Verification items for the finished model (mm, model axes). A direction names the side the tool comes from. Coordinates: 2 decimals unless noted, no trailing zeros. Write each loop counter-clockwise with the first axis right and the second up, starting at its lowest first coordinate (ties: lowest second). Pieces come first, ordered by that corner, then holes. Notation, with made-up numbers: (-39.75, 71) -> (-20.75, 71) arc R20 ccw to (-20.75, 88) -> close; hole circle Ø3 at (63, 22.25). An arc over 180 degrees is marked (long way). Use CSV: the item, a comma, the result in double quotes.
Autodesk Inventor part; units mm, degrees
ref_plane "YZ Plane" through (0, 0, 0) normal (1, 0, 0) x (0, 1, 0)
ref_plane "XZ Plane" through (0, 0, 0) normal (0, 1, 0) x (-1, 0, 0)
ref_plane "XY Plane" through (0, 0, 0) normal (0, 0, 1) x (1, 0, 0)
sketch "Sketch1 - walls" plane through (0, 0, 0) normal (0, 0, 1) x (1, 0, 0)
  line L0 (0, -9) -> (0, 9) construction
  line L1 (-10, -9) -> (-10, -12)
  line L2 (-10, -12) -> (10, -12)
  line L3 (-10, -9) -> (10, -9)
  line L4 (10, -9) -> (10, -12)
  line L5 (-10, 9) -> (10, 9)
  line L6 (10, 9) -> (10, 12)
  line L7 (10, 12) -> (-10, 12)
  line L8 (-10, 12) -> (-10, 9)
  point P0 (0, 0)
  dimension "d5" = 18
  dimension "d7" = 3
  dimension "d8" = 20
  dimension "d9" = 3
  dimension "d10" = 20
extrude "Extrusion1" add sketch "Sketch1 - walls" along normal blind 25
sketch "Sketch2 - base" plane through (0, 0, 0) normal (0, 0, -1) x (-1, 0, 0)
  circle A0 centre (0, 0) radius 18.5
  dimension "d13" = 37
sketch "Sketch3 - wall_top1" plane through (-10, 12, 25) normal (0, 1, 0) x (1, 0, 0)
  line L0 (10, 0) -> (10, -10) construction
  line L1 (20, 0) -> (0, 0)
  arc A0 (0, 0) -> (20, 0) centre (10, 0) ccw
  point P0 (10, 25)
  dimension "d16" = 10
extrude "Extrusion3" add sketch "Sketch3 - wall_top1" against normal blind 3
sketch "Sketch4 - wall_top2" plane through (-10, -12, 25) normal (0, -1, 0) x (1, 0, 0)
  line L0 (10, 0) -> (10, 10) construction
  line L1 (0, 0) -> (20, 0)
  arc A0 (20, 0) -> (0, 0) centre (10, 0) ccw
  dimension "d21" = 10
extrude "Extrusion4" add sketch "Sketch4 - wall_top2" against normal blind 3
extrude "Extrusion2" add sketch "Sketch2 - base" along normal blind 3.5
properties part number "swivel"
1) Set-up check for faces 1 (the flat face through (0, -12, 18)), 2 (the flat face through (0, -9, 18)), 3 (the flat face through (10, 10, 12)): record each of +Z, -Z, +X, -X, +Y, -Y from which the full face is reachable in a straight line by a thin tool's end or side.
Return value:
face 1,"+Z, +X, -X, -Y"
face 2,"+Z, +X, -X"
face 3,"+Z, +X, +Y, -Y"
2) Cross-section at A-A (z = 16.5). Record the boundary of the cut face in (x, y).
Return value:
outline,"(-10, -12) -> (10, -12) -> (10, -9) -> (-10, -9) -> close; (-10, 9) -> (10, 9) -> (10, 12) -> (-10, 12) -> close"
3) Mould release check, pull along Y, two halves, no side actions. Record for faces 4 (the flat face through (0, 12, 17)), 5 (the flat face through (0, 0, -3.5)), 6 (the flat face through (0, 0, 0)): released by +Y, released by -Y, zero draft, split by the parting line, or undercut.
Return value:
face 4,"released by +Y"
face 5,"zero draft"
face 6,"undercut"
4) Cross-section at D-D (x = 6.5). Record the boundary of the cut face in (y, z), plus the area to 3 significant figures.
Return value:
outline,"(-17.32, -3.5) -> (17.32, -3.5) -> (17.32, 0) -> (12, 0) -> (12, 32.6) -> (9, 32.6) -> (9, 0) -> (-9, 0) -> (-9, 32.6) -> (-12, 32.6) -> (-12, 0) -> (-17.32, 0) -> close"
area,"317 mm2"
5) Scan lines: L1, parallel to Y at x = 8, z = 21; L2, parallel to Z at x = 15.5, y = 4.5; L3, parallel to X at y = 11, z = 11. Record each from-to range of solid material in increasing order.
Return value:
L1,"-12 to -9, 9 to 12"
L2,"-3.5 to 0"
L3,"-10 to 10"
6) Cross-section at C-C (y = -6). Record the boundary of the cut face in (x, z), plus the area to 4 significant figures.
Return value:
outline,"(-17.5, -3.5) -> (17.5, -3.5) -> (17.5, 0) -> (-17.5, 0) -> close"
area,"122.5 mm2"
7) Gauge pin test, flat ends, axial feed: pin 1 (8 mm diameter, centred on x = -7.5, y = 7, fed in from +Z); pin 2 (2.5 mm diameter, centred on y = 10, z = 15, fed in from +X); pin 3 (16 mm diameter, centred on x = 2, z = 13.5, fed in from +Y); pin 4 (12 mm diameter, centred on y = 0, z = 28.5, fed in from -X). Record the tip position at first contact, or that the pin passes through.
Return value:
pin 1,"z = 34.15"
pin 2,"x = 10"
pin 3,"y = 12"
pin 4,"through"
8) Cross-section at B-B (x = 0). Record the boundary of the cut face in (y, z).
Return value:
outline,"(-18.5, -3.5) -> (18.5, -3.5) -> (18.5, 0) -> (12, 0) -> (12, 35) -> (9, 35) -> (9, 0) -> (-9, 0) -> (-9, 35) -> (-12, 35) -> (-12, 0) -> (-18.5, 0) -> close"
